Design review of the part shown in the three views and the two pictorial views. Dimensions are in mm from the part's minimum x, y and z. Round coordinates to 2 decimals unless told otherwise and drop trailing zeros. Write each loop counter-clockwise with the first axis right and the second up, starting at its lowest first coordinate (ties: lowest second). Pieces come first, ordered by that corner, then holes. Notation, with made-up numbers: (44, -25) - (50, -25) arc R16 ccw to (50, -21) - close; hole circle Ø9 at (49.5, 89.25). An arc over 180 degrees is marked (long way). One line per item, written item: value. Start each with the question number.
Q1. Add section A-A on z = 5. Write out the cut boundary in (x, y).
Q2. Add section C-C on y = 5.1. Write out the cut boundary in (x, z), and give its area (3 significant figures).
Q3. Mouldability with a two-part tool opening along X and no side actions: class the marked faces 1, 2 and 3 as +X half, -X half, draft (parallel to the pull), parting line (faces both ways), or undercut.
Q4. Add section B-B on x = 36.5. Write out the cut boundary in (y, z).
Q5. Clearance check with flat-ended pins moving along their axes: pin 1 Ø2 at (y, z) = (4, 2) entering from -X; pin 2 Ø3 at (x, z) = (35.61, 5) entering from +Y. State where each tip first meets the part, or that it passes through.
Q6. For probe 1 along X at (y, z) = (2.95, 5); probe 2 along Z at (x, y) = (3, 4.45) (1 decimal); probe 3 along Z at (x, y) = (34.5, 0.6), list the stretches that pass through material, from the lowest coordinate up.
Q7. Add section D-D on z = 1.25. Write out the cut boundary in (x, y), and give its area (3 significant figures).
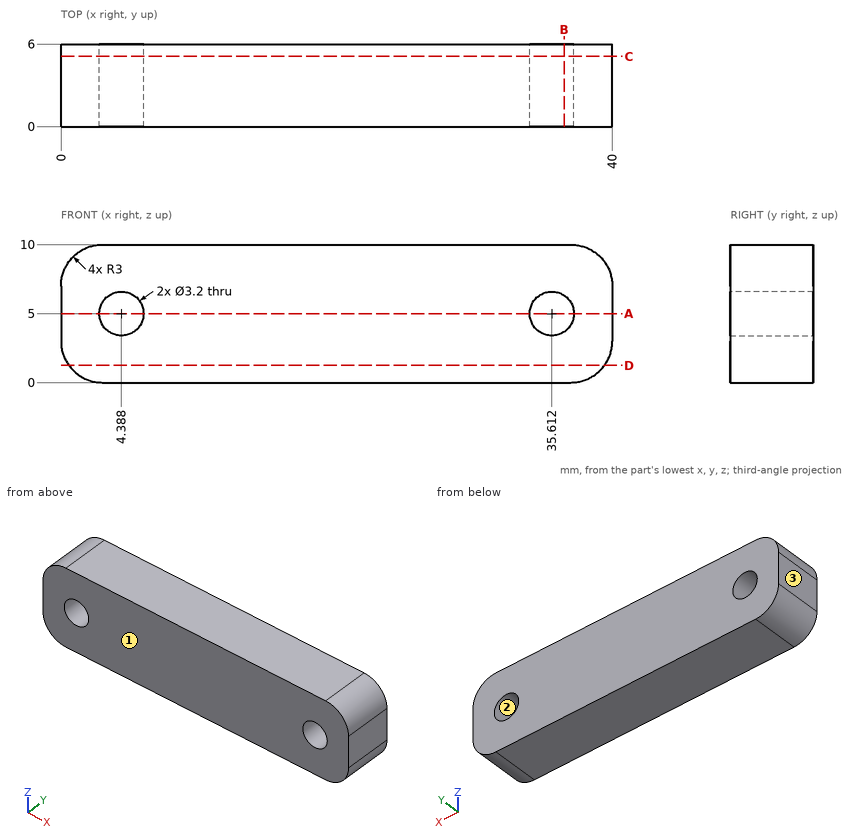
Result set:
1. outline: (0, 0) - (2.79, 0) - (2.79, 6) - (0, 6) - close; (5.99, 0) - (34.01, 0) - (34.01, 6) - (5.99, 6) - close; (37.21, 0) - (40, 0) - (40, 6) - (37.21, 6) - close
2. outline: (0, 3) arc R3 ccw to (3, 0) - (37, 0) arc R3 ccw to (40, 3) - (40, 7) arc R3 ccw to (37, 10) - (3, 10) arc R3 ccw to (0, 7) - close; hole circle Ø3.2 at (4.39, 5); hole circle Ø3.2 at (35.61, 5)
2. area: 376 mm^2
3. face 1: draft
3. face 2: undercut
3. face 3: -X half
4. outline: (0, 0) - (6, 0) - (6, 3.67) - (0, 3.67) - close; (0, 6.33) - (6, 6.33) - (6, 10) - (0, 10) - close
5. pin 1: stops at x = 0
5. pin 2: passes through
6. probe 1: x = 0 to 2.79, 5.99 to 34.01, 37.21 to 40
6. probe 2: z = 0 to 4.2, 5.8 to 10
6. probe 3: z = 0 to 3.85, 6.15 to 10
7. outline: (0.56, 0) - (39.44, 0) - (39.44, 6) - (0.56, 6) - close
7. area: 233 mm^2
